Source: CAD feature listing. Evaluate the final solid. Frame: model axes, mm. A direction names the side the tool comes from. Round coordinates to 2 decimals unless told otherwise and drop trailing zeros. Write each loop counter-clockwise with the first axis right and the second up, starting at its lowest first coordinate (ties: lowest second). Pieces come first, ordered by that corner, then holes.
from build123d import *

# Parameters (mm, degrees)
EXTRUDE_3_DEPTH     = 35
SKETCH_3_R          = 2.1
CUT_EXTRUDE_1_DEPTH = 58.676762411
SKETCH_4_R          = 2.1
CUT_EXTRUDE_2_DEPTH = 58.676762411


with BuildPart() as part:
    # 草图1 → 凸台-拉伸3 (new body)
    with BuildSketch(Plane.XY):
        Polygon((0, 0), (34.154700538, 0), (34.154700538, 2), (1.154700538, 2), (-15.345299462, 30.578838325), (-17.077350269, 29.578838325), align=None)
    extrude(amount=EXTRUDE_3_DEPTH)

    # 草图3 → 切除-拉伸1 (cut, through all)
    with BuildSketch(Plane.XZ):
        with Locations((21.5, 27.5)):
            Circle(SKETCH_3_R)
        with Locations((21.5, 7.5)):
            Circle(SKETCH_3_R)
    extrude(amount=-CUT_EXTRUDE_1_DEPTH, mode=Mode.SUBTRACT)

    # 草图4 → 切除-拉伸2 (cut, through all)
    with BuildSketch(Plane(origin=(0, 0, 0), x_dir=(0, 0, 1), z_dir=(-0.8660254037844397, -0.499999999999998, 0))):
        with Locations(Location((27.5, 20.07, 0), (0, 0, 270))):
            Circle(SKETCH_4_R)
        with Locations(Location((7.5, 20.07, 0), (0, 0, 270))):
            Circle(SKETCH_4_R)
    extrude(amount=-CUT_EXTRUDE_2_DEPTH, mode=Mode.SUBTRACT)


solid = part.part
1) Section query B-B on x = 21.5. Return the cut outline in (y, z), then the cut area to 3 significant figures.
Taken from the geometry:
outline: (0, 0) - (2, 0) - (2, 5.4) - (0, 5.4) - close; (0, 9.6) - (2, 9.6) - (2, 25.4) - (0, 25.4) - close; (0, 29.6) - (2, 29.6) - (2, 35) - (0, 35) - close
area: 53.2 mm2
2) Material intervals for line 1 (Z direction, x = 21.5, y = 1.55); line 2 (Z direction, x = 21, y = 1); line 3 (Y direction, x = 21, z = 17), sorted ascending.
Taken from the geometry:
line 1: z = 0 to 5.4, 9.6 to 25.4, 29.6 to 35
line 2: z = 0 to 5.46, 9.54 to 25.46, 29.54 to 35
line 3: y = 0 to 2
3) Section query D-D on z = 3. Return the cut outline in (x, y), then the cut area to 3 significant figures.
Taken from the geometry:
outline: (-17.08, 29.58) - (0, 0) - (34.15, 0) - (34.15, 2) - (1.15, 2) - (-15.35, 30.58) - close
area: 134 mm2
4) Pull-direction query (X, two-part tool) for faces 3 (the face through (22.63, 0.99, 9.27)), 4 (the face through (-6.98, 16.09, 17.26)), 5 (the face through (23.503, 0.986, 28.131)), 6 (the face through (4.6, 1.8, 0)); classes: released by +X, released by -X, zero draft, split by the parting line, or undercut.
Taken from the geometry:
face 3: undercut
face 4: released by +X
face 5: undercut
face 6: zero draft
5) Contact query for flat-ended pins moving along their axis: P1, Ø5, axis at x = -4.5, z = 13, coming from the -Y side; P2, Ø5, axis at x = 25.5, z = 5, coming from the +Y side; P3, Ø4, axis at y = 22, z = 26.5, coming from the +X side. Output: stop coordinate, or through.
Taken from the geometry:
P1: stops at y = 3.46
P2: stops at y = 2
P3: stops at x = -9.24
6) Reachability of faces 1 (the face through (18, 2, 17)), 2 (the face through (-9.318, 18.111, 9.582)) from +Z, -Z, +X, -X, +Y, -Y: full face, straight path, thin tool, end or side. Return the list, or none.
Taken from the geometry:
face 1: +Z, -Z, +X, +Y
face 2: none
7) Section query C-C on x = 8. Return the cut outline in (y, z).
Taken from the geometry:
outline: (0, 0) - (2, 0) - (2, 35) - (0, 35) - close
8) Section query A-A on z = 27.5. Return the cut outline in (x, y) (3 decimals).
Taken from the geometry:
outline: (-17.077, 29.579) - (-11.085, 19.2) - (-9.353, 20.2) - (-15.345, 30.579) - close; (-8.985, 15.562) - (0, 0) - (19.4, 0) - (19.4, 2) - (1.155, 2) - (-7.253, 16.562) - close; (23.6, 0) - (34.155, 0) - (34.155, 2) - (23.6, 2) - close
